Geometry check sheet. Reference: the model listing, model coordinates, mm. A direction names the side the tool comes from. Give positions to 0.01 mm unless a question says otherwise; leave off trailing zeros. Loops run counter-clockwise (first coordinate to the right, second up) from the corner with the lowest first, then second, coordinate; pieces in that order, holes last.
```python
from build123d import *

# Parameters (mm, degrees)
F0_W     = 30
F0_H     = 20
F1_DEPTH = 8
F2_R     = 8.25
F2_R_2   = 5.2
F3_DEPTH = 8
F4_R     = 1.75
F4_R_2   = 5.2
F5_DEPTH = 25
F6_R     = 5


with BuildPart() as f1:
    # F0 (on Top) → F1 (new body)
    with BuildSketch(Plane.XY):
        with Locations((15, 10)):
            Rectangle(F0_W, F0_H)
    extrude(amount=F1_DEPTH)

    # F2 (on face) → F3 (join)
    with BuildSketch(Plane.XY.offset(8)):
        with Locations((15, 10)):
            Circle(F2_R)
        with Locations((15, 10)):
            Circle(F2_R_2, mode=Mode.SUBTRACT)
    extrude(amount=F3_DEPTH)

    # F4 (on face) → F5 (cut)
    with BuildSketch(Plane.XY.offset(8)):
        with Locations((3.5, 10)):
            Circle(F4_R)
        with Locations((26.5, 10)):
            Circle(F4_R)
        with Locations((15, 10)):
            Circle(F4_R_2)
    extrude(amount=-F5_DEPTH, mode=Mode.SUBTRACT)

    # F6
    f6_edges = [f1.edges().sort_by_distance(p)[0] for p in [
        (0, 0, 4),
        (30, 0, 4),
        (30, 20, 4),
        (0, 20, 4),
    ]]
    fillet(f6_edges, radius=F6_R)


solid = f1.part
```
1) Scan lines: line 1 along Y through (x, z) = (15, 3.75); line 2 along Y through (x, z) = (15, 13.5); line 3 along X through (y, z) = (9.75, 3.25). Record each from-to range of solid material in increasing order.
2) Sectioned sample at A-A on y = 10. Enter the section's corners in (x, z), plus the area to 3 significant figures.
3) Depth check by flat-ended pin: P1, Ø1, axis at y = 17, z = 4.5, coming from the -X side; P2, Ø1.5, axis at x = 26, z = 9, coming from the -Y side; P3, Ø2, axis at x = 14.5, z = 11.5, coming from the +Y side; P4, Ø5.5, axis at x = 26.5, y = 10, coming from the +Z side. Enter the tip coordinate at first touch or a pass-through.
4) Sectioned sample at C-C on z = 4.25. Enter the section's corners in (x, y).
5) Tool access check on faces 1 (the cylindrical face through (18.807, 2.681, 11.944)), 2 (the flat face through (30, 10, 4)). Record the directions out of +Z, -Z, +X, -X, +Y, -Y that give a thin tool (end or side, any length) a straight path to the whole face; none if there is none.
6) Sectioned sample at B-B on x = 15. Enter the section's corners in (y, z).
7) Mould release check, pull along X, two halves, no side actions. Record for faces 3 (the cylindrical face through (24.75, 10.08, 4.06)), 4 (the flat face through (11, 6, 0)), 5 (the flat face through (0, 10, 4)): +X half, -X half, draft (parallel to the pull), parting line (faces both ways), or undercut.
8) Sectioned sample at D-D on y = 5.5. Enter the section's corners in (x, z), plus the area to 3 significant figures.
Determined:
1. line 1: y = 0 to 4.8, 15.2 to 20
1. line 2: y = 1.75 to 4.8, 15.2 to 18.25
1. line 3: x = 0 to 1.77, 5.23 to 9.81, 20.19 to 24.77, 28.23 to 30
2. outline: (0, 0) - (1.75, 0) - (1.75, 8) - (0, 8) - close; (5.25, 0) - (9.8, 0) - (9.8, 16) - (6.75, 16) - (6.75, 8) - (5.25, 8) - close; (20.2, 0) - (24.75, 0) - (24.75, 8) - (23.25, 8) - (23.25, 16) - (20.2, 16) - close; (28.25, 0) - (30, 0) - (30, 8) - (28.25, 8) - close
2. area: 150 mm2
3. P1: stops at x = 0.23
3. P2: passes through
3. P3: stops at y = 18.25
3. P4: stops at z = 8
4. outline: (0, 5) arc R5 ccw to (5, 0) - (25, 0) arc R5 ccw to (30, 5) - (30, 15) arc R5 ccw to (25, 20) - (5, 20) arc R5 ccw to (0, 15) - close; hole circle Ø3.5 at (3.5, 10); hole circle Ø10.4 at (15, 10); hole circle Ø3.5 at (26.5, 10)
5. face 1: +Z
5. face 2: +Z, -Z, +X, +Y, -Y
6. outline: (0, 0) - (4.8, 0) - (4.8, 16) - (1.75, 16) - (1.75, 8) - (0, 8) - close; (15.2, 0) - (20, 0) - (20, 8) - (18.25, 8) - (18.25, 16) - (15.2, 16) - close
7. face 3: undercut
7. face 4: draft
7. face 5: -X half
8. outline: (0, 0) - (12.39, 0) - (12.39, 16) - (8.09, 16) - (8.09, 8) - (0, 8) - close; (17.61, 0) - (30, 0) - (30, 8) - (21.91, 8) - (21.91, 16) - (17.61, 16) - close
8. area: 267 mm2
